Verification items for this drawing (mm, ordinates from the low corner). A direction names the side the tool comes from. Coordinates: 2 decimals unless noted, no trailing zeros. Order: outer loops, then holes, each group sorted by start corner. A loop starts at its lowest first (then second) coordinate and runs counter-clockwise, first axis right, second up.
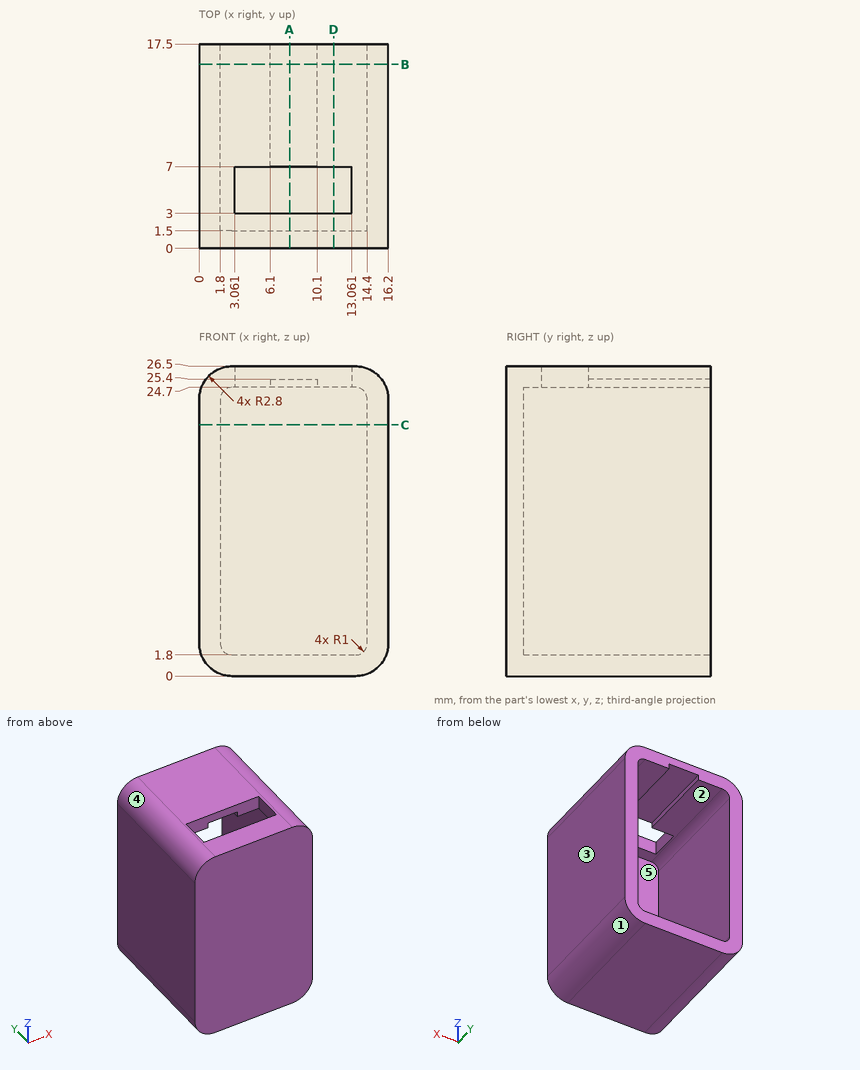
(1) Cross-section at A-A (x = 7.75). Enter the section's corners in (y, z), and give its area (3 significant figures).
Filled in:
outline: (0, 0) - (17.5, 0) - (17.5, 1.8) - (1.5, 1.8) - (1.5, 24.7) - (3, 24.7) - (3, 26.5) - (0, 26.5) - close; (7, 25.4) - (17.5, 25.4) - (17.5, 26.5) - (7, 26.5) - close
area: 82.8 mm2
(2) Release check for a two-part mould opening along X. For the marked faces 3, 4 and 5 record: +X half, -X half, draft (parallel to the pull), parting line (faces both ways), or undercut.
Filled in:
face 3: +X half
face 4: -X half
face 5: undercut
(3) Thickness scan on probe 1 along Z at (x, y) = (12.5, 16.75); probe 2 along X at (y, z) = (5.25, 16); probe 3 along Z at (x, y) = (8.25, 9.5). Record the ranges inside material, lowest first.
Filled in:
probe 1: z = 0 to 1.8, 24.7 to 26.5
probe 2: x = 0 to 1.8, 14.4 to 16.2
probe 3: z = 0 to 1.8, 25.4 to 26.5
(4) Cross-section at B-B (y = 15.75). Enter the section's corners in (x, z), and give its area (3 significant figures).
Filled in:
outline: (0, 2.8) arc R2.8 ccw to (2.8, 0) - (13.4, 0) arc R2.8 ccw to (16.2, 2.8) - (16.2, 23.7) arc R2.8 ccw to (13.4, 26.5) - (2.8, 26.5) arc R2.8 ccw to (0, 23.7) - close; hole (1.8, 2.8) arc R1 ccw to (2.8, 1.8) - (13.4, 1.8) arc R1 ccw to (14.4, 2.8) - (14.4, 23.7) arc R1 ccw to (13.4, 24.7) - (10.1, 24.7) - (10.1, 25.4) - (6.1, 25.4) - (6.1, 24.7) - (2.8, 24.7) arc R1 ccw to (1.8, 23.7) - close
area: 132 mm2
(5) Cross-section at D-D (x = 11.5). Enter the section's corners in (y, z).
Filled in:
outline: (0, 0) - (17.5, 0) - (17.5, 1.8) - (1.5, 1.8) - (1.5, 24.7) - (3, 24.7) - (3, 26.5) - (0, 26.5) - close; (7, 24.7) - (17.5, 24.7) - (17.5, 26.5) - (7, 26.5) - close
(6) Tool access check on the marked faces 1 and 2. Record the directions out of +Z, -Z, +X, -X, +Y, -Y that give a thin tool (end or side, any length) a straight path to the whole face; none if there is none.
Filled in:
face 1: -Z, +X, +Y, -Y
face 2: +Y
(7) Cross-section at C-C (z = 21.5). Enter the section's corners in (x, y).
Filled in:
outline: (0, 0) - (16.2, 0) - (16.2, 17.5) - (14.4, 17.5) - (14.4, 1.5) - (1.8, 1.5) - (1.8, 17.5) - (0, 17.5) - close
(8) Go/stop test with flat-tipped pins: P1, Ø6, axis at x = 11, y = 8, coming from the -Z side; P2, Ø2, axis at y = 5, z = 26, coming from the +X side; P3, Ø0.5, axis at y = 5, z = 25.5, coming from the -X side; P4, Ø0.8, axis at y = 11.5, z = 25, coming from the -X side. Record where each tip stops, or that it passes through.
Filled in:
P1: stops at z = 0
P2: stops at x = 15.88
P3: stops at x = 0.47
P4: stops at x = 0.15
